The figure shows three views and two pictorial views of one solid part (mm, origin at its lowest corner). Answer the questions. A direction names the side the tool comes from. Give positions to 0.01 mm unless a question says otherwise; leave off trailing zeros. Write each loop counter-clockwise with the first axis right and the second up, starting at its lowest first coordinate (ties: lowest second). Pieces come first, ordered by that corner, then holes. Notation, with made-up numbers: (-31, -2.5) - (-27, -2.5) arc R31 cw to (-27, 24.5) - close; hole circle Ø6 at (-39, 30.25). An arc over 180 degrees is marked (long way). Write each question's results on one line, items separated by ' | '. Start each with the question number.
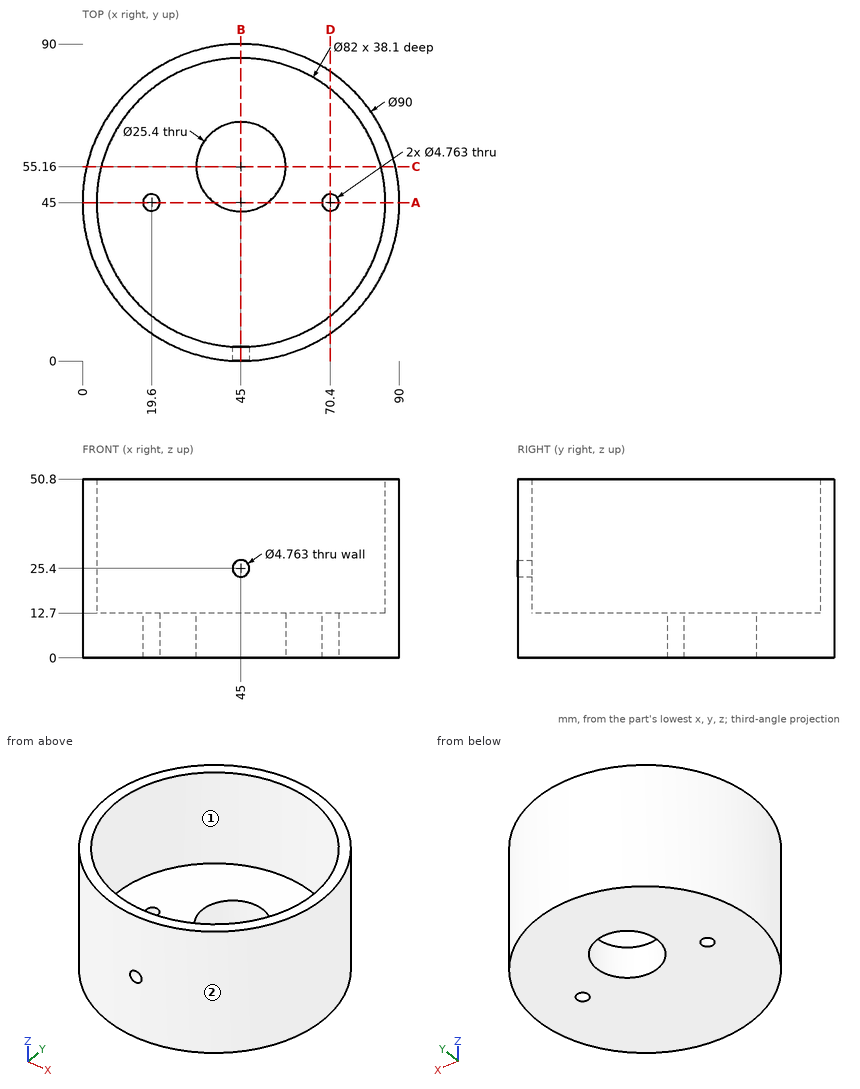
Q1. A cutting plane is placed at D-D, the plane x = 70.4. Write down the section's boundary in (y, z) (1 decimal).
Q2. A cutting plane is placed at A-A, the plane y = 45. Write down the section's boundary in (x, z), and give its area (3 significant figures).
Q3. A tool of negligible diameter and unlimited length cuts with its end or side. For the marked faces 1 and 2, from which of +Z, -Z, +X, -X, +Y, -Y can it reach the whole face along a straight path? Write none if from no direction.
Q4. A cutting plane is placed at C-C, the plane y = 55.16. Write down the section's boundary in (x, z), and give its area (3 significant figures).
Q5. Given pin 1 (6 mm diameter, centred on x = 38, y = 44, fed in from +Z); pin 2 (12 mm diameter, centred on x = 21.5, z = 40.5, fed in from -Y); pin 3 (15 mm diameter, centred on x = 45, y = 55.16, fed in from +Z); pin 4 (2 mm diameter, centred on x = 59.5, z = 27.5, fed in from +Y), each flat-ended and moving along its own axis, determine where each tip first touches the part or whether it passes through.
Q6. A cutting plane is placed at B-B, the plane x = 45. Write down the section's boundary in (y, z).
Q7. Consider L1, parallel to Y at x = 45, z = 7.75; L2, parallel to Z at x = 72.5, y = 69; L3, parallel to X at y = 72, z = 19.5 (1 decimal). Determine where each line is inside the solid, lowest interval first.
Result:
1) outline: (7.9, 0) - (42.6, 0) - (42.6, 12.7) - (12.8, 12.7) - (12.8, 50.8) - (7.9, 50.8) - close; (47.4, 0) - (82.1, 0) - (82.1, 50.8) - (77.2, 50.8) - (77.2, 12.7) - (47.4, 12.7) - close
2) outline: (0, 0) - (17.22, 0) - (17.22, 12.7) - (4, 12.7) - (4, 50.8) - (0, 50.8) - close; (21.98, 0) - (37.38, 0) - (37.38, 12.7) - (21.98, 12.7) - close; (52.62, 0) - (68.02, 0) - (68.02, 12.7) - (52.62, 12.7) - close; (72.78, 0) - (90, 0) - (90, 50.8) - (86, 50.8) - (86, 12.7) - (72.78, 12.7) - close | area: 1,130 mm2
3) face 1: +Z | face 2: +Z, -Z
4) outline: (1.16, 0) - (32.3, 0) - (32.3, 12.7) - (5.28, 12.7) - (5.28, 50.8) - (1.16, 50.8) - close; (57.7, 0) - (88.84, 0) - (88.84, 50.8) - (84.72, 50.8) - (84.72, 12.7) - (57.7, 12.7) - close | area: 1,100 mm2
5) pin 1: stops at z = 12.7 | pin 2: stops at y = 3.54 | pin 3: passes through | pin 4: stops at y = 87.93
6) outline: (0, 0) - (42.46, 0) - (42.46, 12.7) - (4, 12.7) - (4, 23.02) - (0, 23.02) - close; (0, 27.78) - (4, 27.78) - (4, 50.8) - (0, 50.8) - close; (67.86, 0) - (90, 0) - (90, 50.8) - (86, 50.8) - (86, 12.7) - (67.86, 12.7) - close
7) L1: y = 0 to 42.46, 67.86 to 90 | L2: z = 0 to 12.7 | L3: x = 9 to 14.1, 75.9 to 81
